```python
from build123d import *

# Parameters (mm, degrees)
SKIZZE1_R          = 72.5
SKIZZE1_R_2        = 72
COVER_RING_DEPTH   = 25.5
SKIZZE2_R          = 1.5
SPACER_SCREW_DEPTH = 1
KREISMUSTER1_COUNT = 4


with BuildPart() as part:
    # Skizze1 → Cover Ring (new body)
    with BuildSketch(Plane.XY):
        Circle(SKIZZE1_R)
        Circle(SKIZZE1_R_2, mode=Mode.SUBTRACT)
    extrude(amount=COVER_RING_DEPTH)

    # Skizze2 → Spacer Screw (add)
    with BuildSketch(Plane.XY):
        with BuildLine():
            Line((48.790367902, 53.033008589), (45.608387387, 49.851028074))
            ThreePointArc((45.608387387, 49.851028074), (45.608387387, 45.608387387), (49.851028074, 45.608387387))
            Line((49.851028074, 45.608387387), (53.033008589, 48.790367902))
            Line((53.033008589, 48.790367902), (48.790367902, 53.033008589))
        make_face()
        with Locations((47.72970773, 47.72970773)):
            Circle(SKIZZE2_R, mode=Mode.SUBTRACT)
    spacer_screw = extrude(amount=SPACER_SCREW_DEPTH)

    # Kreismuster1: Spacer Screw ×4 about axis
    kreismuster1_axis = Axis((0, 0, 0), (0, 0, 1))
    for i in range(1, KREISMUSTER1_COUNT):
        add(spacer_screw.rotate(kreismuster1_axis, i * 360 / KREISMUSTER1_COUNT))


solid = part.part
```
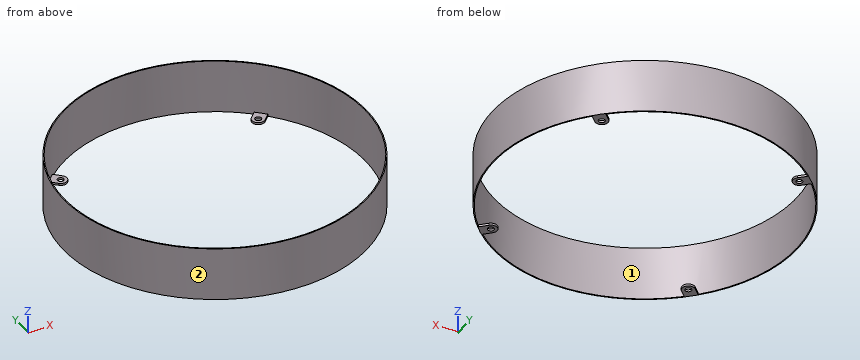
Build history of the part. All positions in model axes, mm. Face numbers are marked on the shaded views. Give positions to 0.01 mm unless a question says otherwise; leave off trailing zeros. Order: outer loops, then holes, each group sorted by start corner. A loop starts at its lowest first (then second) coordinate and runs counter-clockwise, first axis right, second up. Notation, with made-up numbers: M 58.25,44.5 L 68.25,44.5 A19 ccw 68.25,71.5 Z; hole C 26.5,-12 d8. An arc over 180 degrees is marked long. Return JSON: item names as keys, results as strings.
Q1. Wall check: probe 1 along Y at (x, z) = (0, 6); probe 2 along X at (y, z) = (-1.5, 9); probe 3 along Y at (x, z) = (-17, 17.5). Give the ranges that are in metal, low to high. Write a range as from..to.
Answer list:
{"probe 1": "y = -72.5..-72, 72..72.5", "probe 2": "x = -72.48..-71.98, 71.98..72.48", "probe 3": "y = -70.48..-69.96, 69.96..70.48"}
Q2. Band-saw the part on B-B (y = 0). Give the cut face in (x, z).
Answer list:
{"outline": "M -72.5,0 L -72,0 L -72,25.5 L -72.5,25.5 Z; M 72,0 L 72.5,0 L 72.5,25.5 L 72,25.5 Z"}
Q3. Band-saw the part on C-C (z = 17). Give the cut face in (x, y), then the cut area to 3 significant figures.
Answer list:
{"outline": "C 0,0 d145; hole C 0,0 d144", "area": "227 mm^2"}
Q4. Two-plate mould, pull along X, no slides. Class the marked faces 1 and 2: pulls with the +X half, pulls with the -X half, needs draft (parallel to the pull), parting line crosses it, or undercut.
Answer list:
{"face 1": "undercut", "face 2": "parting line crosses it"}
Q5. Flat gauge pins, fed straight in: pin 1 (12 mm diameter, centred on y = 39, z = 6, fed in from -X); pin 2 (2 mm diameter, centred on x = 8.5, z = 23, fed in from -Y); pin 3 (2.5 mm diameter, centred on x = -48.5, y = 50, fed in from +Z). Where does each tip first touch, or does it go through?
Answer list:
{"pin 1": "stops at x = -64.55", "pin 2": "stops at y = -72.11", "pin 3": "stops at z = 1"}
